from build123d import *

# Parameters (mm, degrees)
SKETCH1_R           = 0.5
BOSS_EXTRUDE1_DEPTH = 3
CUT_EXTRUDE2_DEPTH  = 65.730209331


with BuildPart() as part:
    # Sketch1 → Boss-Extrude1 (new body)
    with BuildSketch(Plane.XY):
        with BuildLine():
            Line((-5, 0), (5, 0))
            Line((5, 0), (5, 3))
            Line((5, 3), (21, 3))
            Line((21, 3), (21, 0))
            Line((21, 0), (26, 0))
            Line((26, 0), (26, 3))
            Line((26, 3), (40, 3))
            ThreePointArc((40, 3), (44.043458593, 7.866487724), (50, 10))
            Line((50, 10), (50, 21))
            Line((50, 21), (55, 21))
            Line((55, 21), (55, 31))
            Line((55, 31), (50, 31))
            Line((50, 31), (50, 34))
            Line((50, 34), (0, 34))
            Line((0, 34), (-50, 34))
            Line((-50, 34), (-50, 31))
            Line((-50, 31), (-55, 31))
            Line((-55, 31), (-55, 21))
            Line((-55, 21), (-50, 21))
            Line((-50, 21), (-50, 10))
            Line((-50, 10), (-40, 3))
            Line((-40, 3), (-26, 3))
            Line((-26, 3), (-26, 0))
            Line((-26, 0), (-21, 0))
            Line((-21, 0), (-21, 3))
            Line((-21, 3), (-5, 3))
            Line((-5, 3), (-5, 0))
        make_face()
        with Locations((28, 32)):
            Circle(SKETCH1_R, mode=Mode.SUBTRACT)
        with Locations((28, 20.7)):
            Circle(SKETCH1_R, mode=Mode.SUBTRACT)
        with Locations(Location((-28, 20.7, 0), (0, 0, 180))):
            Circle(SKETCH1_R, mode=Mode.SUBTRACT)
        with Locations(Location((-28, 32, 0), (0, 0, 180))):
            Circle(SKETCH1_R, mode=Mode.SUBTRACT)
    extrude(amount=BOSS_EXTRUDE1_DEPTH)

    # Sketch3 → Cut-Extrude2 (cut, through all)
    with BuildSketch(Plane.XY.offset(3)):
        with BuildLine():
            Line((-50, 32), (-50, 31))
            ThreePointArc((-50, 31), (-49.5, 31.5), (-50, 32))
        make_face()
        with BuildLine():
            ThreePointArc((-50, 20), (-49.5, 20.5), (-50, 21))
            Line((-50, 21), (-50, 20))
        make_face()
        with BuildLine():
            Line((-27, 3), (-26, 3))
            ThreePointArc((-26, 3), (-26.5, 3.5), (-27, 3))
        make_face()
        with BuildLine():
            ThreePointArc((-20, 3), (-20.5, 3.5), (-21, 3))
            Line((-21, 3), (-20, 3))
        make_face()
        with BuildLine():
            ThreePointArc((-5, 3), (-5.5, 3.5), (-6, 3))
            Line((-6, 3), (-5, 3))
        make_face()
        with BuildLine():
            ThreePointArc((6, 3), (5.5, 3.5), (5, 3))
            Line((5, 3), (6, 3))
        make_face()
        with BuildLine():
            ThreePointArc((21, 3), (20.5, 3.5), (20, 3))
            Line((20, 3), (21, 3))
        make_face()
        with BuildLine():
            ThreePointArc((27, 3), (26.5, 3.5), (26, 3))
            Line((26, 3), (27, 3))
        make_face()
        with BuildLine():
            Line((50, 20), (50, 21))
            ThreePointArc((50, 21), (49.5, 20.5), (50, 20))
        make_face()
        with BuildLine():
            ThreePointArc((50, 32), (49.5, 31.5), (50, 31))
            Line((50, 31), (50, 32))
        make_face()
    extrude(amount=-CUT_EXTRUDE2_DEPTH, mode=Mode.SUBTRACT)


solid = part.part
Could you check a few things on this model? Use its own coordinates, in mm. A direction names the side the tool comes from. Give positions to 0.01 mm unless a question says otherwise; leave off trailing zeros. Write each loop counter-clockwise with the first axis right and the second up, starting at its lowest first coordinate (ties: lowest second). Pieces come first, ordered by that corner, then holes. Notation, with made-up numbers: (56.5, -18.75) -> (90.5, -18.75) arc R16 ccw to (90.5, -1.75) -> close; hole circle Ø4 at (-39.75, -28.5). An arc over 180 degrees is marked (long way). Write each question's results on one line, items separated by ' | '. Start each with the question number.
Q1. Suppose I cut it at B-B, the plane x = -38.5. List the corners of the cut face in (y, z) for me.
Q2. Suppose I cut it at C-C, the plane z = 1.35. State how many separate pieces and enclosed holes the cut face has, and give its area (3 significant figures).
Q3. Which directions (+Z, -Z, +X, -X, +Y, -Y) give clear straight access to the entire face, cutting with the end or side of a thin tool? Please do faces 1 (the face through (53, 31, 1)), 2 (the face through (-26, 2, 1)), 3 (the face through (-52, 31, 1)).
Q4. We'd pull the mould along X, two halves only. Please class faces 4 (the face through (-34, 3, 1)), 5 (the face through (50, 15, 1)), 6 (the face through (21, 2, 1)), 7 (the face through (-50, 15, 1)): +X half, -X half, draft (parallel to the pull), parting line (faces both ways), or undercut.
Q5. Suppose I cut it at A-A, the plane y = 11.5. List the corners of the cut face in (x, z) for me.
Q6. I need wall thicknesses on probe 1 along Y at (x, z) = (-28, 1.2); probe 2 along Y at (x, z) = (14, 2.05); probe 3 along X at (y, z) = (15, 2.35). Which ranges of each line are inside material? Lowest first, please.
Q7. I'm going to push flat-ended pins straight in: pin 1 Ø0.9 at (x, z) = (-52.5, 2) entering from +Y; pin 2 Ø0.9 at (x, z) = (-52, 1.5) entering from -Y; pin 3 Ø1.5 at (x, z) = (13, 1) entering from -Y; pin 4 Ø1 at (x, z) = (-4, 2) entering from -Y. Where does each tip first touch, or does it pass through?
Outcome:
1) outline: (3, 0) -> (34, 0) -> (34, 3) -> (3, 3) -> close
2) separate pieces: 1 | enclosed holes: 4 | area: 3,170 mm2
3) face 1: +Z, -Z, +X, +Y | face 2: +Z, -Z, -X, -Y | face 3: +Z, -Z, -X, +Y
4) face 4: draft | face 5: +X half | face 6: undercut | face 7: -X half
5) outline: (-50, 0) -> (50, 0) -> (50, 3) -> (-50, 3) -> close
6) probe 1: 3 to 20.2, 21.2 to 31.5, 32.5 to 34 | probe 2: 3 to 34 | probe 3: -50 to 50
7) pin 1: y = 31 | pin 2: y = 21 | pin 3: y = 3 | pin 4: y = 0
